CAD build for the part. Positions are in the model's coordinates, mm. A direction names the side the tool comes from. Round coordinates to 2 decimals unless told otherwise and drop trailing zeros. Loops run counter-clockwise (first coordinate to the right, second up) from the corner with the lowest first, then second, coordinate; pieces in that order, holes last.
```python
from build123d import *

# Parameters (mm, degrees)
BOSS_EXTRUDE1_DEPTH = 30
SKETCH2_R           = 2.25
CUT_EXTRUDE1_DEPTH  = 57.77507973
SKETCH3_R           = 5
CUT_EXTRUDE2_DEPTH  = 54.530698882
FILLET1_R           = 3


with BuildPart() as part:
    # Sketch1 → Boss-Extrude1 (new body)
    with BuildSketch(Plane(origin=(0, 0, 0), x_dir=(1, 0, 0), z_dir=(0, 1, 0))):
        Polygon((3.5, -15), (32.5, 15), (-32.5, 15), (-32.5, -15), align=None)
    extrude(amount=BOSS_EXTRUDE1_DEPTH)

    # Sketch2 → Cut-Extrude1 (cut, through all)
    with BuildSketch(Plane(origin=(9.304997128, 0, 8.994830557), x_dir=(0.6950220968474751, 0, -0.7189883760491118), z_dir=(0.7189883760491118, 0, 0.6950220968474751))):
        with Locations((18.623043788, 15)):
            Circle(SKETCH2_R)
        with Locations((1.123043788, 15)):
            Circle(SKETCH2_R)
    extrude(amount=-CUT_EXTRUDE1_DEPTH, mode=Mode.SUBTRACT)

    # Sketch3 → Cut-Extrude2 (cut, through all)
    with BuildSketch(Plane(origin=(6.429043624, 0, 6.21474217), x_dir=(0.6950220968474751, 0, -0.7189883760491118), z_dir=(0.7189883760491118, 0, 0.6950220968474751))):
        with Locations((18.623043788, 15)):
            Circle(SKETCH3_R)
        with Locations((1.123043788, 15)):
            Circle(SKETCH3_R)
    extrude(amount=-CUT_EXTRUDE2_DEPTH, mode=Mode.SUBTRACT)

    # Fillet1
    fillet1_edges = [part.edges().sort_by_distance(p)[0] for p in [
        (-14.5, 30, 15),
        (0, 30, -15),
        (-14.5, 0, 15),
        (-32.5, 0, 0),
        (0, 0, -15),
        (-32.5, 30, 0),
        (-32.5, 15, 15),
        (-32.5, 15, -15),
    ]]
    fillet(fillet1_edges, radius=FILLET1_R)


solid = part.part
```
Item 1: Cut at B-B, the plane z = -12.75. State how many separate pieces and enclosed holes the cut face has, plus the area to 3 significant figures.
Answers follow:
separate pieces: 1
enclosed holes: 2
area: 1,640 mm2
Item 2: Cut at A-A, the plane y = 23. Give the cut face in (x, z), plus the area to 3 significant figures.
Answers follow:
outline: (-32.5, -12) arc R3 ccw to (-29.5, -15) - (32.5, -15) - (3.5, 15) - (-29.5, 15) arc R3 ccw to (-32.5, 12) - close
area: 1,510 mm2
Item 3: Probe line 1 (X direction, y = 18.25, z = -9.5); line 2 (X direction, y = 14, z = -9.5); line 3 (X direction, y = 16.5, z = 0.25). List the from-to ranges inside material, lowest first.
Answers follow:
line 1: x = -32.5 to -13.68, -2.74 to 11.5, 21.62 to 27.18
line 2: x = -32.5 to -15.26, -1.16 to 9.92, 21.62 to 27.18
line 3: x = -32.5 to -4.99, 8.74 to 17.76
Item 4: Two-plate mould, pull along Y, no slides. Class faces 3 (the flat face through (6.389, 12.848, 6.256)), 4 (the cylindrical face through (-5.8, 15.22, -0.22)), 5 (the cylindrical face through (1.07, 0.86, -14.1)), 6 (the flat face through (-32.5, 15, 0)): released by +Y, released by -Y, zero draft, split by the parting line, or undercut.
Answers follow:
face 3: undercut
face 4: undercut
face 5: released by -Y
face 6: zero draft
Item 5: Cut at C-C, the plane y = 11.5. Give the cut face in (x, z), plus the area to 3 significant figures.
Answers follow:
outline: (-32.5, -12) arc R3 ccw to (-29.5, -15) - (-19.04, -15) - (4.73, 7.97) - (9.69, 2.84) - (-8.76, -15) - (6.14, -15) - (16.89, -4.61) - (21.85, -9.74) - (16.42, -15) - (32.5, -15) - (3.5, 15) - (-29.5, 15) arc R3 ccw to (-32.5, 12) - close
area: 1,220 mm2
Item 6: 3-axis set-ups, long thin cutter, end or side, ignore diameter. For faces 1 (the flat face through (-13, 15, 15)), 2 (the flat face through (18.552, 12.848, -6.326)): which of +Z, -Z, +X, -X, +Y, -Y reach the whole face in a straight line?
Answers follow:
face 1: +Z, +X, -X, +Y, -Y
face 2: none
Item 7: Flat gauge pins, fed straight in: P1, Ø6, axis at y = 18, z = 7, coming from the +X side; P2, Ø2, axis at y = 22, z = 3, coming from the +X side; P3, Ø5, axis at y = 10, z = -2, coming from the +X side. Where does each tip first touch, or does it go through?
Answers follow:
P1: stops at x = 14.13
P2: stops at x = 16.07
P3: stops at x = 22.35
